The model under review builds one solid part; all positions refer to its coordinate system, in mm. A direction names the side the tool comes from. Give positions to 0.01 mm unless a question says otherwise; leave off trailing zeros. Loops run counter-clockwise (first coordinate to the right, second up) from the corner with the lowest first, then second, coordinate; pieces in that order, holes last. Notation, with made-up numbers: (-17, 43) - (1, 43) arc R33 cw to (1, 79) - close; hole circle Ø11 at (-27, 51.5). An arc over 180 degrees is marked (long way). Answer as a JSON object with one key per item and string values.
from build123d import *

# Parameters (mm, degrees)
SKETCH_1_R             = 18.5
EXTRUDE_1_DEPTH        = 24
SKETCH_2_R             = 17
EXTRUDE_2_DEPTH        = 22
SKETCH_3_R             = 3
SKETCH_3_W             = 0.5
SKETCH_3_H             = 3
EXTRUDE_3_DEPTH        = 3
SKETCH_4_R             = 17
EXTRUDE_4_DEPTH        = 1.5
SKETCH_5_R             = 7
EXTRUDE_5_DEPTH        = 5
SKETCH_6_W             = 1
SKETCH_6_H             = 4
EXTRUDE_6_DEPTH        = 2
SKETCH_7_W             = 16
SKETCH_7_H             = 6
EXTRUDE_7_DEPTH        = 5
SKETCH_8_W             = 14
SKETCH_8_H             = 4
EXTRUDE_8_DEPTH        = 2.5
SKETCH_9_R             = 0.5
EXTRUDE_9_DEPTH        = 10
PATTERN_LINEAR_1_COUNT = 6
PATTERN_LINEAR_1_PITCH = 2
SKETCH_11_R            = 5.5
EXTRUDE_10_DEPTH       = 5.5
EXTRUDE_11_DEPTH       = 15
CUT_EXTRUDE_2_DEPTH    = 0.4
SKETCH_14_R            = 2
CUT_EXTRUDE_3_DEPTH    = 0.5
SKETCH_15_R            = 2
CUT_EXTRUDE_4_DEPTH    = 3


with BuildPart() as part:
    # 草图1 → 凸台-拉伸1 (new body)
    with BuildSketch(Plane.XY):
        Circle(SKETCH_1_R)
    extrude(amount=EXTRUDE_1_DEPTH)

    # 草图2 → 凸台-拉伸2 (add)
    with BuildSketch(Plane.XY.offset(24)):
        Circle(SKETCH_2_R)
    extrude(amount=EXTRUDE_2_DEPTH)

    # 草图3 → 凸台-拉伸3 (add)
    with BuildSketch(Plane.XY.offset(46)):
        Circle(SKETCH_3_R)
        with Locations((-12.75, 0)):
            Rectangle(SKETCH_3_W, SKETCH_3_H)
        with Locations((12.75, 0)):
            Rectangle(SKETCH_3_W, SKETCH_3_H)
    extrude(amount=EXTRUDE_3_DEPTH)

    # 草图4 → 凸台-拉伸4 (add)
    with BuildSketch(Plane.XY.offset(49)):
        Circle(SKETCH_4_R)
    extrude(amount=EXTRUDE_4_DEPTH)

    # 草图5 → 凸台-拉伸5 (add)
    with BuildSketch(Plane.XY.offset(50.5)):
        Circle(SKETCH_5_R)
        Polygon((-5.656854249, -5.656854249), (-6.363961031, -4.949747468), (-8.131727984, -5.303300859), (-6.717514421, -6.717514421), (-5.303300859, -8.131727984), (-4.949747468, -6.363961031), align=None)
        Polygon((5.656854249, -5.656854249), (6.363961031, -4.949747468), (8.131727984, -5.303300859), (6.717514421, -6.717514421), (5.303300859, -8.131727984), (4.949747468, -6.363961031), align=None)
    extrude(amount=EXTRUDE_5_DEPTH)

    # 草图6 → 凸台-拉伸6 (add)
    with BuildSketch(Plane.XY.offset(50.5)):
        with Locations((-13, 0)):
            Rectangle(SKETCH_6_W, SKETCH_6_H)
        with Locations((13, 0)):
            Rectangle(SKETCH_6_W, SKETCH_6_H)
    extrude(amount=EXTRUDE_6_DEPTH)

    # 草图7 → 凸台-拉伸7 (add)
    with BuildSketch(Plane.XY.offset(50.5)):
        with Locations((0, 11)):
            Rectangle(SKETCH_7_W, SKETCH_7_H)
    extrude(amount=EXTRUDE_7_DEPTH)

    # 草图8 → 凸台-拉伸8 (add)
    with BuildSketch(Plane(origin=(0, 14, 0), x_dir=(1, 0, 0), z_dir=(0, 1, 0))):
        with Locations((0, -52.7)):
            Rectangle(SKETCH_8_W, SKETCH_8_H)
    extrude(amount=EXTRUDE_8_DEPTH)

    # 草图9 → 凸台-拉伸9 (add)
    with BuildSketch(Plane(origin=(0, 16.5, 0), x_dir=(1, 0, 0), z_dir=(0, 1, 0))):
        with Locations(Location((5, -52.95, 0), (0, 0, 270))):
            Circle(SKETCH_9_R)
    extrude_9 = extrude(amount=EXTRUDE_9_DEPTH)

    # 阵列(线性)1: 凸台-拉伸9 ×6
    with Locations(*[(-i * PATTERN_LINEAR_1_PITCH, 0, 0) for i in range(1, PATTERN_LINEAR_1_COUNT)]):
        add(extrude_9)

    # 草图11 → 凸台-拉伸10 (add)
    with BuildSketch(Plane(origin=(0, 0, 0), x_dir=(-1, 0, 0), z_dir=(0, 0, -1))):
        with Locations((7.498333348, -0.158104393)):
            Circle(SKETCH_11_R)
    extrude(amount=EXTRUDE_10_DEPTH)

    # 草图12 → 凸台-拉伸11 (add)
    with BuildSketch(Plane(origin=(0, 0, -5.5), x_dir=(-1, 0, 0), z_dir=(0, 0, -1))):
        with BuildLine():
            Line((5.262265371, 1.841895607), (9.734401326, 1.841895607))
            ThreePointArc((9.734401326, 1.841895607), (7.498333348, -3.158104393), (5.262265371, 1.841895607))
        make_face()
    extrude(amount=EXTRUDE_11_DEPTH)

    # 草图10 → 切除-拉伸2 (cut)
    with BuildSketch(Plane(origin=(0, 0, 0), x_dir=(-1, 0, 0), z_dir=(0, 0, -1))):
        with BuildLine():
            ThreePointArc((10.036531252, 6.36551051), (-11.882294081, 0.250541395), (9.759293221, -6.78291084))
            ThreePointArc((9.759293221, -6.78291084), (0.49988889, -0.010540293), (10.036531252, 6.36551051))
        make_face()
    extrude(amount=-CUT_EXTRUDE_2_DEPTH, mode=Mode.SUBTRACT)

    # 草图14 → 切除-拉伸3 (cut)
    with BuildSketch(Plane(origin=(0, 0, 0), x_dir=(-1, 0, 0), z_dir=(0, 0, -1))):
        with Locations((8.039373582, 13.833599402)):
            Circle(SKETCH_14_R)
        with Locations((7.449117181, -14.160178432)):
            Circle(SKETCH_14_R)
        with Locations((-15.996444476, 0.337289372)):
            Circle(SKETCH_14_R)
    extrude(amount=-CUT_EXTRUDE_3_DEPTH, mode=Mode.SUBTRACT)

    # 草图15 → 切除-拉伸4 (cut)
    with BuildSketch(Plane(origin=(0, 0, 0), x_dir=(-1, 0, 0), z_dir=(0, 0, -1))):
        with Locations((-0.337289372, -15.996444476)):
            Circle(SKETCH_15_R)
        with Locations((0.337289372, 15.996444476)):
            Circle(SKETCH_15_R)
        with Locations((-14.021971973, -7.706121074)):
            Circle(SKETCH_15_R)
        with Locations((-13.684682601, 8.290323403)):
            Circle(SKETCH_15_R)
        with Locations((13.684682601, -8.290323403)):
            Circle(SKETCH_15_R)
        with Locations((14.021971973, 7.706121074)):
            Circle(SKETCH_15_R)
    extrude(amount=-CUT_EXTRUDE_4_DEPTH, mode=Mode.SUBTRACT)


solid = part.part
Q1. To check wall thickness, follow probe 1 along Z at (x, y) = (-9, 6.5); probe 2 along Z at (x, y) = (-5.5, 12); probe 3 along Z at (x, y) = (-12, 13.5). State the ranges of each line that lie inside material, in increasing order. Write a range as [from, to].
Results:
{"probe 1": "z = [0, 46], [49, 50.5]", "probe 2": "z = [0, 46], [49, 55.5]", "probe 3": "z = [0, 24]"}
Q2. Clearance check with flat-ended pins moving along their axes: pin 1 Ø10 at (y, z) = (14, 37) entering from +X; pin 2 Ø6 at (y, z) = (-3.5, 13.5) entering from +X; pin 3 Ø6 at (x, y) = (5, -10.5) entering from -Z. State where each tip first meets the part, or that it passes through.
Results:
{"pin 1": "stops at x = 14.42", "pin 2": "stops at x = 18.49", "pin 3": "stops at z = 0"}
Q3. For faces 1 (the face through (5.13, -7.26, 52.96)), 2 (the face through (-13.5, 0, 51)), 3 (the face through (6.466, -2.681, 52.965)), 4 (the face through (-8, 11, 53)), 5 (the face through (-0.08, 17.98, 1.48)), list the 3-axis set-ups (+Z, -Z, +X, -X, +Y, -Y) from which the entire face can be reached by the end or side of a thin tool; tool diameter is ignored.
Results:
{"face 1": "+Z, -Y", "face 2": "+Z, -X, +Y, -Y", "face 3": "+Z", "face 4": "+Z, -X, +Y", "face 5": "-Z"}
Q4. Consider section B-B, the plane z = 2. State the section outline as (x, y) points.
Results:
{"outline": "circle Ø37 at (0, 0); hole circle Ø4 at (-14.02, 7.71); hole circle Ø4 at (-13.68, -8.29); hole circle Ø4 at (-0.34, 16); hole circle Ø4 at (0.34, -16); hole circle Ø4 at (13.68, 8.29); hole circle Ø4 at (14.02, -7.71)"}
Q5. The part is to be moulded in two halves that separate along Z. For faces 6 (the face through (-12.5, 0, 47)), 7 (the face through (12.5, 0, 51)), 8 (the face through (6, -6, 55.5)), say which applies: +Z half, -Z half, draft (parallel to the pull), parting line (faces both ways), or undercut.
Results:
{"face 6": "undercut", "face 7": "draft", "face 8": "+Z half"}
Q6. Consider section C-C, the plane z = 42. State the section outline as (x, y) points, plus the area to 3 significant figures.
Results:
{"outline": "circle Ø34 at (0, 0)", "area": "908 mm^2"}
Q7. Consider section A-A, the plane y = 20. State the section outline as (x, z) points, plus the area to 3 significant figures.
Results:
{"outline": "circle Ø1 at (-5, 52.95); circle Ø1 at (-3, 52.95); circle Ø1 at (-1, 52.95); circle Ø1 at (1, 52.95); circle Ø1 at (3, 52.95); circle Ø1 at (5, 52.95)", "area": "4.71 mm^2"}
